Autodesk Inventor part; units mm, degrees
ref_plane "YZ Plane" through (0, 0, 0) normal (1, 0, 0) x (0, 1, 0)
ref_plane "XZ Plane" through (0, 0, 0) normal (0, 1, 0) x (-1, 0, 0)
ref_plane "XY Plane" through (0, 0, 0) normal (0, 0, 1) x (1, 0, 0)
sketch "スケッチ1" plane through (0, 0, 0) normal (0, 0, 1) x (1, 0, 0)
  line L0 (-31.5, 11.5) -> (31.5, 11.5)
  line L1 (31.5, 11.5) -> (31.5, -11.5)
  line L2 (31.5, -11.5) -> (-31.5, -11.5)
  line L3 (-31.5, -11.5) -> (-31.5, 11.5)
  line L4 (-31.5, 11.5) -> (31.5, -11.5) construction
  line L5 (31.5, 11.5) -> (-31.5, -11.5) construction
  line L6 (-30, 10) -> (30, 10) construction
  line L7 (30, 10) -> (30, -10) construction
  line L8 (30, -10) -> (-30, -10) construction
  line L9 (-30, -10) -> (-30, 10) construction
  line L10 (-30, 10) -> (30, -10) construction
  line L11 (30, 10) -> (-30, -10) construction
  circle A0 centre (-28, 8) radius 1.25
  line L12 (-31.5, 0) -> (31.5, 0) construction
  line L13 (0, 11.5) -> (0, -11.5) construction
  circle A1 centre (-28, -8) radius 1.25
  circle A2 centre (28, 8) radius 1.25
  circle A3 centre (28, -8) radius 1.25
  line L14 (-30.25, 10.25) -> (30.25, 10.25)
  line L15 (30.25, 10.25) -> (30.25, -10.25)
  line L16 (30.25, -10.25) -> (-30.25, -10.25)
  line L17 (-30.25, -10.25) -> (-30.25, 10.25)
  line L18 (-30.25, 10.25) -> (30.25, -10.25) construction
  line L19 (30.25, 10.25) -> (-30.25, -10.25) construction
  line L20 (-21.92, 9) -> (-3.92, 9)
  line L21 (-3.92, 9) -> (-3.92, -9)
  line L22 (-3.92, -9) -> (-21.92, -9)
  line L23 (-21.92, -9) -> (-21.92, 9)
  line L24 (-21.92, 9) -> (-3.92, -9) construction
  line L25 (-3.92, 9) -> (-21.92, -9) construction
  line L26 (21.92, 9) -> (3.92, 9)
  line L27 (3.92, 9) -> (3.92, -9)
  line L28 (3.92, -9) -> (21.92, -9)
  line L29 (21.92, -9) -> (21.92, 9)
  line L30 (21.92, 9) -> (3.92, -9) construction
  line L31 (3.92, 9) -> (21.92, -9) construction
  arc A4 (-30.25, 6.9103) -> (-26.9103, 10.25) centre (-28, 8) ccw
  arc A5 (-26.9103, -10.25) -> (-30.25, -6.9103) centre (-28, -8) ccw
  arc A6 (26.9103, 10.25) -> (30.25, 6.9103) centre (28, 8) ccw
  arc A7 (30.25, -6.9103) -> (26.9103, -10.25) centre (28, -8) ccw
  line L32 (30.25, 5) -> (31.5, 5)
  line L33 (30.25, -5) -> (31.5, -5)
  point P0 (0, 0)
  point P1 (0, 0)
  point P2 (-12.92, 0)
  point P3 (12.92, 0)
  point P4 (30.25, -6.9103)
  point P5 (26.9103, -10.25)
  point P6 (-30.25, -6.9103)
  point P7 (30.25, 6.9103)
  dimension "d0" = 63
  dimension "d1" = 60
  dimension "d2" = 20
  dimension "d3" = 23
  dimension "d4" = 2.5
  dimension "d5" = 2
  dimension "d6" = 2
  dimension "d7" = 20.5
  dimension "d8" = 60.5
  dimension "d17" = 18
  dimension "d18" = 18
  dimension "d19" = 17.08
  dimension "d22" = 2.5
  dimension "d23" = 10
extrude "押し出し1" add sketch "スケッチ1" against normal blind 2
extrude "押し出し5" add sketch "スケッチ1" along normal blind 3 contours L0 L1 L32 L15 L14 L17 L16 L33 L2 L3 | A6 L14 L15 | L15 L16 A7 | A4 L17 L14 | L16 L17 A5
fillet "フィレット2" radius 1 12 edges at (-31.5, 11.5, 0.5) (-31.5, -11.5, 0.5) (31.5, -11.5, 0.5) (31.5, 11.5, 0.5) (26.9103, 10.25, 1.5) (30.25, 6.9103, 1.5) (30.25, -6.9103, 1.5) (26.9103, -10.25, 1.5) (-26.9103, -10.25, 1.5) (-30.25, -6.9103, 1.5) (-30.25, 6.9103, 1.5) (-26.9103, 10.25, 1.5)
equation "\"d6\" = d5"
equation "\"d17\" = d18"
properties part number "StartStopSwitch_cover_01" material "アセタール樹脂、黒"
The model under review builds one solid part; all positions refer to its coordinate system, in mm. A direction names the side the tool comes from. Give positions to 0.01 mm unless a question says otherwise; leave off trailing zeros. Write each loop counter-clockwise with the first axis right and the second up, starting at its lowest first coordinate (ties: lowest second). Pieces come first, ordered by that corner, then holes.
(1) For P1, Ø12, axis at x = 18, y = 0.5, coming from the -Z side; P2, Ø2.5, axis at y = 1.5, z = 2, coming from the +X side, all flat-tipped, find the tip position at first contact; note any pin that passes through.
(2) Tool access review of faces 1 (the flat face through (-21.92, 0, -1)), 2 (the flat face through (0, -11.5, 1)), 3 (the cylindrical face through (-29.828, 5.547, 1.479)): name each direction out of +Z, -Z, +X, -X, +Y, -Y from which nothing blocks a thin tool from reaching the whole face with its end or side.
(3) Consider section A-A, the plane y = 4. Give the boundary of the cut face in (x, z), and give its area (4 significant figures).
(4) Consider section B-B, the plane z = -0.6. Give the boundary of the cut face in (x, y).
(5) The part is to be moulded in two halves that separate along X. For faces 4 (the flat face through (-30.25, 0, 1)), 5 (the cylindrical face through (25.56, -9.81, 1.48)), 6 (the flat face through (-5, 11, 3)), say which applies: released by +X, released by -X, zero draft, split by the parting line, or undercut.
(6) Consider section C-C, the plane x = -28. Give the boundary of the cut face in (y, z).
(7) To check wall thickness, follow L1, parallel to Y at x = -28, z = -0.1; L2, parallel to Y at x = 28, z = 2.05; L3, parallel to Y at x = 16, z = -0.9. State the ranges of each line that lie inside material, in increasing order.
(8) Consider section D-D, the plane x = 11. Give the boundary of the cut face in (y, z), and give its area (3 significant figures).
Returned:
1. P1: stops at z = -2
1. P2: stops at x = -30.25
2. face 1: +Z, -Z
2. face 2: +Z, -Z, +X, -X, -Y
2. face 3: +Z
3. outline: (-31.5, -2) - (-21.92, -2) - (-21.92, 0) - (-30.25, 0) - (-30.25, 3) - (-31.5, 3) - close; (-3.92, -2) - (3.92, -2) - (3.92, 0) - (-3.92, 0) - close; (21.92, -2) - (31.5, -2) - (31.5, 0) - (21.92, 0) - close
3. area: 57.75 mm2
4. outline: (-31.5, -10.5) arc R1 ccw to (-30.5, -11.5) - (30.5, -11.5) arc R1 ccw to (31.5, -10.5) - (31.5, 10.5) arc R1 ccw to (30.5, 11.5) - (-30.5, 11.5) arc R1 ccw to (-31.5, 10.5) - close; hole circle Ø2.5 at (-28, -8); hole circle Ø2.5 at (-28, 8); hole (-21.92, -9) - (-3.92, -9) - (-3.92, 9) - (-21.92, 9) - close; hole (3.92, -9) - (21.92, -9) - (21.92, 9) - (3.92, 9) - close; hole circle Ø2.5 at (28, -8); hole circle Ø2.5 at (28, 8)
5. face 4: released by +X
5. face 5: undercut
5. face 6: zero draft
6. outline: (-11.5, -2) - (-9.25, -2) - (-9.25, 3) - (-11.5, 3) - close; (-6.75, -2) - (6.75, -2) - (6.75, 3) - (5.5, 3) - (5.5, 0) - (-5.5, 0) - (-5.5, 3) - (-6.75, 3) - close; (9.25, -2) - (11.5, -2) - (11.5, 3) - (9.25, 3) - close
7. L1: y = -11.5 to -9.25, -6.75 to 6.75, 9.25 to 11.5
7. L2: y = -11.5 to -9.25, -6.75 to -5.5, 5.5 to 6.75, 9.25 to 11.5
7. L3: y = -11.5 to -9, 9 to 11.5
8. outline: (-11.5, -2) - (-9, -2) - (-9, 0) - (-10.25, 0) - (-10.25, 3) - (-11.5, 3) - close; (9, -2) - (11.5, -2) - (11.5, 3) - (10.25, 3) - (10.25, 0) - (9, 0) - close
8. area: 17.5 mm2
